Input: part model. Units: mm. Frame: model coordinates. Face numbers are marked on the shaded views. A direction names the side the tool comes from. Round coordinates to 2 decimals unless told otherwise and drop trailing zeros. Loops run counter-clockwise (first coordinate to the right, second up) from the corner with the lowest first, then second, coordinate; pieces in that order, holes last.
1) First-contact query: pin 1 (8 mm diameter, centred on y = 11, z = 10, fed in from -X); pin 2 (8 mm diameter, centred on x = 6.5, y = 5, fed in from -Z); pin 3 (6 mm diameter, centred on x = 30.5, y = 12, fed in from -Z). Flat tips, straight axial feed; report the tip coordinate or a pass-through.
2) Ray query, line 1 along X through (y, z) = (8.5, 0); line 2 along X through (y, z) = (12, 31); line 3 along Z through (x, y) = (28, 8). Return the intervals inside material, ascending.
3) Draft query along Z for the marked faces 1 and 2. Return one class per face: pulls with the +Z half, pulls with the -Z half, needs draft (parallel to the pull), parting line crosses it, or undercut.
4) Section A-A, the plane y = 6.5. State how many separate pieces and enclosed holes the cut face has, and give its area (3 significant figures).
5) Access query for the marked faces 3 and 4. Directions: +Z, -Z, +X, -X, +Y, -Y. A direction counts if a zero-diameter tool reaches every point of the face in a straight line with its end or side. Return the directions, or none.
6) Section B-B, the plane x = 0. Return loops of the section in (y, z), and give its area (4 significant figures).
from build123d import *

# Parameters (mm, degrees)
ESBO_O1_W             = 19.9
ESBO_O1_H             = 15
ESBO_O2_R             = 4.65
CORTE_EXTRUS_O1_DEPTH = 69.415495321
CORTE_EXTRUS_O2_DEPTH = 69.415495321
CHANFRO1_SIZE         = 1
CHANFRO2_SIZE         = 1
CHANFRO3_SIZE         = 1
CHANFRO4_SIZE         = 1


with BuildPart() as part:
    # Esboço1 → Revolução1 (revolve)
    with BuildSketch(Plane.XY, mode=Mode.PRIVATE) as revolu_o1_sk:
        with Locations((37.25, 7.5)):
            Rectangle(ESBO_O1_W, ESBO_O1_H)
    revolve(revolu_o1_sk.sketch.rotate(Axis((0, -49.922822823, 0), (0, 1, 0)), 90), axis=Axis((0, -49.922822823, 0), (0, 1, 0)))

    # Esboço2 → Corte-extrusão1 (cut, through all)
    with BuildSketch(Plane(origin=(0, 15, 0), x_dir=(1, 0, 0), z_dir=(0, 1, 0))):
        with Locations(Location((-39.5, 0, 0), (0, 0, 270))):
            Circle(ESBO_O2_R)
        with Locations(Location((-19.75, 34.208003449, 0), (0, 0, 270))):
            Circle(ESBO_O2_R)
        with Locations(Location((19.75, 34.208003449, 0), (0, 0, 270))):
            Circle(ESBO_O2_R)
        with Locations(Location((39.5, 0, 0), (0, 0, 270))):
            Circle(ESBO_O2_R)
        with Locations(Location((19.75, -34.208003449, 0), (0, 0, 270))):
            Circle(ESBO_O2_R)
        with Locations(Location((-19.75, -34.208003449, 0), (0, 0, 270))):
            Circle(ESBO_O2_R)
    extrude(amount=-CORTE_EXTRUS_O1_DEPTH, mode=Mode.SUBTRACT)

    # Esboço3 → Corte-extrusão2 (cut, through all)
    with BuildSketch(Plane(origin=(0, 15, 0), x_dir=(1, 0, 0), z_dir=(0, 1, 0))):
        with BuildLine():
            Line((5.25, 34.654581227), (7.355, 26.290568176))
            ThreePointArc((7.355, 26.290568176), (0, 27.3), (-7.355, 26.290568176))
            Line((-7.355, 26.290568176), (-5.25, 34.654581227))
            ThreePointArc((-5.25, 34.654581227), (0, 35.05), (5.25, 34.654581227))
        make_face()
        with BuildLine():
            Line((32.6367477, 12.780657243), (26.44579992, 6.775667243))
            ThreePointArc((26.44579992, 6.775667243), (23.642493523, 13.65), (19.09079992, 19.514900933))
            Line((19.09079992, 19.514900933), (27.3867477, 21.873923983))
            ThreePointArc((27.3867477, 21.873923983), (30.354190403, 17.525), (32.6367477, 12.780657243))
        make_face()
        with BuildLine():
            Line((27.3867477, -21.873923983), (19.09079992, -19.514900933))
            ThreePointArc((19.09079992, -19.514900933), (23.642493523, -13.65), (26.44579992, -6.775667243))
            Line((26.44579992, -6.775667243), (32.6367477, -12.780657243))
            ThreePointArc((32.6367477, -12.780657243), (30.354190403, -17.525), (27.3867477, -21.873923983))
        make_face()
        with BuildLine():
            Line((-5.25, -34.654581227), (-7.355, -26.290568176))
            ThreePointArc((-7.355, -26.290568176), (0, -27.3), (7.355, -26.290568176))
            Line((7.355, -26.290568176), (5.25, -34.654581227))
            ThreePointArc((5.25, -34.654581227), (0, -35.05), (-5.25, -34.654581227))
        make_face()
        with BuildLine():
            Line((-32.6367477, -12.780657243), (-26.44579992, -6.775667243))
            ThreePointArc((-26.44579992, -6.775667243), (-23.642493523, -13.65), (-19.09079992, -19.514900933))
            Line((-19.09079992, -19.514900933), (-27.3867477, -21.873923983))
            ThreePointArc((-27.3867477, -21.873923983), (-30.354190403, -17.525), (-32.6367477, -12.780657243))
        make_face()
        with BuildLine():
            Line((-27.3867477, 21.873923983), (-19.09079992, 19.514900933))
            ThreePointArc((-19.09079992, 19.514900933), (-23.642493523, 13.65), (-26.44579992, 6.775667243))
            Line((-26.44579992, 6.775667243), (-32.6367477, 12.780657243))
            ThreePointArc((-32.6367477, 12.780657243), (-30.354190403, 17.525), (-27.3867477, 21.873923983))
        make_face()
    extrude(amount=-CORTE_EXTRUS_O2_DEPTH, mode=Mode.SUBTRACT)

    # Chanfro1
    chanfro1_edges = [part.edges().sort_by_distance(p)[0] for p in [
        (-13.65, 0, -23.642493523),
        (-13.65, 15, -23.642493523),
        (0, 0, 47.2),
        (0, 15, 47.2),
        (13.65, 15, -23.642493523),
        (27.3, 15, 0),
        (13.65, 15, 23.642493523),
        (-13.65, 15, 23.642493523),
        (-27.3, 0, 0),
        (-27.3, 15, 0),
    ]]
    chamfer(chanfro1_edges, length=CHANFRO1_SIZE)

    # Chanfro2
    chanfro2_edges = [part.edges().sort_by_distance(p)[0] for p in [
        (13.65, 0, -23.642493523),
        (27.3, 0, 0),
        (13.65, 0, 23.642493523),
        (-13.65, 0, 23.642493523),
    ]]
    chamfer(chanfro2_edges, length=CHANFRO2_SIZE)

    # Chanfro3
    chanfro3_edges = [part.edges().sort_by_distance(p)[0] for p in [
        (-39.5, 0, -4.65),
        (-19.75, 0, -38.858003449),
        (19.75, 0, -38.858003449),
        (39.5, 0, -4.65),
        (19.75, 0, 29.558003449),
        (-19.75, 0, 29.558003449),
    ]]
    chamfer(chanfro3_edges, length=CHANFRO3_SIZE)

    # Chanfro4
    chanfro4_edges = [part.edges().sort_by_distance(p)[0] for p in [
        (-39.5, 15, -4.65),
        (-19.75, 15, -38.858003449),
        (19.75, 15, -38.858003449),
        (39.5, 15, -4.65),
        (19.75, 15, 29.558003449),
        (-19.75, 15, 29.558003449),
    ]]
    chamfer(chanfro4_edges, length=CHANFRO4_SIZE)


solid = part.part
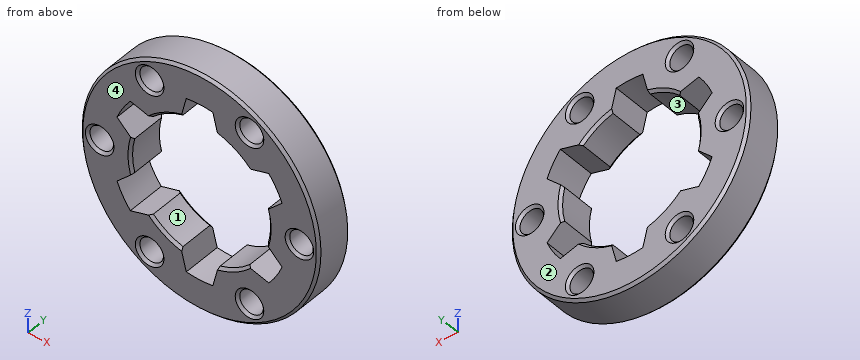
Final values:
1. pin 1: stops at x = -46.82
1. pin 2: stops at z = -47.13
1. pin 3: stops at z = -38.36
2. line 1: x = -47.2 to -44.15, -34.85 to -27.3, 27.3 to 34.85, 44.15 to 47.2
2. line 2: x = -35.59 to -23.12, -16.38 to -6.17, 6.17 to 16.38, 23.12 to 35.59
2. line 3: z = -38 to -21.08, -8.28 to 8.28, 21.08 to 38
3. face 1: undercut
3. face 2: needs draft
4. separate pieces: 1
4. enclosed holes: 7
4. area: 3,660 mm2
5. face 3: +Y, -Y
5. face 4: +Z, -Z, +X, -X, -Y
6. outline: (0, -46.2) - (1, -47.2) - (14, -47.2) - (15, -46.2) - (15, -35.05) - (0, -35.05) - close; (0, 35.05) - (15, 35.05) - (15, 46.2) - (14, 47.2) - (1, 47.2) - (0, 46.2) - close
6. area: 362.5 mm2
